Source: CAD feature listing. Evaluate the final solid. Frame: model axes, mm. A direction names the side the tool comes from. Give positions to 0.01 mm unless a question says otherwise; leave off trailing zeros. Order: outer loops, then holes, each group sorted by start corner. A loop starts at its lowest first (then second) coordinate and runs counter-clockwise, first axis right, second up. Notation, with made-up numbers: (-22.75, 73.25) -> (-15.75, 73.25) arc R27 cw to (-15.75, 110.25) -> close; hole circle Ø7 at (5.5, -8). An arc over 180 degrees is marked (long way). Use CSV: the item, a comma, the result in double quotes.
```python
from build123d import *

# Parameters (mm, degrees)
F0_R           = 50
F1_DEPTH       = 2
F3_R           = 10
F4_DEPTH       = 1.5
F5_D           = 6.4
F5_CSINK_D     = 13.44
F5_CSINK_ANGLE = 90


with BuildPart() as f1:
    # F0 (on Top) → F1 (new body)
    with BuildSketch(Plane.XY):
        Circle(F0_R)
    extrude(amount=F1_DEPTH)

    # F3 (on face) → F4 (join)
    with BuildSketch(Plane(origin=(0, 0, 0), x_dir=(1, 0, 0), z_dir=(0, 0, -1))):
        with Locations((31.9376476109, 0)):
            Circle(F3_R)
        with Locations((-32.1291722357, 0)):
            Circle(F3_R)
    extrude(amount=F4_DEPTH)

    # F5 (through all)
    with Locations(Plane.XY.offset(2)):
        with Locations((-32, 0), (32, 0)):
            CounterSinkHole(F5_D / 2, F5_CSINK_D / 2, counter_sink_angle=F5_CSINK_ANGLE)


solid = f1.part
```
1. Ray query, line 1 along Y through (x, z) = (30.5, -1.05); line 2 along Z through (x, y) = (-26, 42); line 3 along Y through (x, z) = (-28, 1.35). Return the intervals inside material, ascending.
Answer below:
line 1,"y = -9.9 to -3.35, 3.35 to 9.9"
line 2,"z = 0 to 2"
line 3,"y = -41.42 to -4.57, 4.57 to 41.42"
2. Pin query (flat end, axial travel): P1, Ø1, axis at x = 36, z = 1.5, coming from the -Y side; P2, Ø12, axis at x = 18, y = 20, coming from the -Z side. Return the tip coordinate at first contact, or that it passes through.
Answer below:
P1,"stops at y = -35.21"
P2,"stops at z = 0"
3. Section query C-C on x = 0. Return loops of the section in (y, z).
Answer below:
outline,"(-50, 0) -> (50, 0) -> (50, 2) -> (-50, 2) -> close"
4. Access query for faces 1 (the flat face through (-34.5, -2.4, -1.5)), 2 (the cylindrical face through (-42.12, -0.44, -0.74)). Directions: +Z, -Z, +X, -X, +Y, -Y. A direction counts if a zero-diameter tool reaches every point of the face in a straight line with its end or side. Return the directions, or none.
Answer below:
face 1,"-Z, +X, -X, +Y, -Y"
face 2,"-Z"
5. Section query B-B on x = -32. Return loops of the section in (y, z), plus the area to 3 significant figures.
Answer below:
outline,"(-38.42, 0) -> (-10, 0) -> (-10, -1.5) -> (-3.22, -1.5) -> (-6.72, 2) -> (-38.42, 2) -> close; (3.22, -1.5) -> (10, -1.5) -> (10, 0) -> (38.42, 0) -> (38.42, 2) -> (6.72, 2) -> close"
area,"149 mm²"
6. Section query A-A on y = 0. Return loops of the section in (x, z).
Answer below:
outline,"(-50, 0) -> (-42.13, 0) -> (-42.13, -1.5) -> (-35.22, -1.5) -> (-38.72, 2) -> (-50, 2) -> close; (-28.78, -1.5) -> (-22.13, -1.5) -> (-22.13, 0) -> (21.94, 0) -> (21.94, -1.5) -> (28.78, -1.5) -> (25.28, 2) -> (-25.28, 2) -> close; (35.22, -1.5) -> (41.94, -1.5) -> (41.94, 0) -> (50, 0) -> (50, 2) -> (38.72, 2) -> close"
7. Mould query, pull axis X, two halves, no side actions, for faces 3 (the flat face through (-1, 1, 2)), 4 (the conical face through (-35.23, 1.02, -1.33)), 5 (the cylindrical face through (47.69, 15.02, 0.99)). Classes: released by +X, released by -X, zero draft, split by the parting line, or undercut.
Answer below:
face 3,"zero draft"
face 4,"undercut"
face 5,"split by the parting line"
